Design review of the part built by this model. Coordinates are the model's own, in mm. Coordinates: 2 decimals unless noted, no trailing zeros. Order: outer loops, then holes, each group sorted by start corner. A loop starts at its lowest first (then second) coordinate and runs counter-clockwise, first axis right, second up. Notation, with made-up numbers: (37.25, 12.25) -> (84.25, 12.25) arc R11 cw to (84.25, 17.25) -> close; hole circle Ø8 at (-8.5, -14.75). An arc over 180 degrees is marked (long way). Use a Markdown table: item, result. Add a question column.
Q1. Insertion check: pin 1 (1.6 mm diameter, centred on x = -52, z = -2.5, fed in from -Y); pin 2 (1.6 mm diameter, centred on y = -15.5, z = -3, fed in from -X); pin 3 (8.5 mm diameter, centred on x = 0, y = 0, fed in from +Z); pin 4 (1.6 mm diameter, centred on x = 40.5, z = -3.5, fed in from +Y). Each pin has a flat end and moves straight along its axis. Give the tip position at first contact, or say it passes through.
Q2. Add section D-D (x = -30). State the section outline as (y, z) points, then the cut area to 3 significant figures.
Q3. Add section B-B (z = -2.9). Count the separate pieces of the cut face and the enclosed holes in it, then the cut area to 3 significant figures.
Q4. Add section A-A (x = 0). State the section outline as (y, z) points, then the cut area to 3 significant figures.
Q5. Wall thickness on probe 1 along X at (y, z) = (0, -3.05); probe 2 along Y at (x, z) = (30, -2.8); probe 3 along X at (y, z) = (21.5, -2.1): over which ranges is each line inside the solid? List them lowest first.
Q6. Add section C-C (y = 0). State the section outline as (x, z) points, then the cut area to 3 significant figures.
Autodesk Inventor part; units mm, degrees
ref_plane "YZ Plane" through (0, 0, 0) normal (1, 0, 0) x (0, 1, 0)
ref_plane "XZ Plane" through (0, 0, 0) normal (0, 1, 0) x (-1, 0, 0)
ref_plane "XY Plane" through (0, 0, 0) normal (0, 0, 1) x (1, 0, 0)
sketch "Block1" plane through (0, 0, 0) normal (0, 0, 1) x (1, 0, 0)
  line L0 (-37.5521, 20) -> (-37.5521, 24)
  line L1 (-37.5521, 24) -> (-17.5521, 24)
  line L2 (-17.5521, 24) -> (-17.5521, 20)
  line L3 (-37.4196, 20) -> (-17.5521, 20)
  line L4 (17.5521, 24) -> (17.5521, 20)
  line L5 (37.5521, 20) -> (37.5521, 24)
  line L6 (37.5521, 24) -> (17.5521, 24)
  line L7 (37.4196, 20) -> (17.5521, 20)
  point P0 (0, 21.8462)
  dimension "d140" = 20
  dimension "d141" = 4
sketch "Block2" plane through (0, 0, 0) normal (0, 0, 1) x (1, 0, 0)
  line L0 (-33.5533, 20.22) -> (-33.5533, 29.22)
  line L1 (-33.5533, 29.22) -> (-13.1133, 29.22)
  line L2 (-13.1133, 29.22) -> (-13.1133, 20.22)
  line L3 (-13.1133, 20.22) -> (13.1133, 20.22)
  line L4 (13.1133, 20.22) -> (13.1133, 29.22)
  line L5 (13.1133, 29.22) -> (33.5533, 29.22)
  line L6 (33.5533, 29.22) -> (33.5533, 20.22)
  line L7 (33.5533, 20.22) -> (50.22, 20.22)
  line L8 (50.22, 20.22) -> (50.22, 13.5533)
  line L9 (50.22, 13.5533) -> (59.22, 13.5533)
  line L10 (59.22, 13.5533) -> (59.22, 5.1133)
  line L11 (59.22, 5.1133) -> (50.22, 5.1133)
  line L12 (50.22, 5.1133) -> (50.22, -5.1133)
  line L13 (50.22, -5.1133) -> (59.22, -5.1133)
  line L14 (59.22, -5.1133) -> (59.22, -13.5533)
  line L15 (59.22, -13.5533) -> (50.22, -13.5533)
  line L16 (50.22, -13.5533) -> (50.22, -20.22)
  line L17 (50.22, -20.22) -> (-50.22, -20.22)
  line L18 (-50.22, -20.22) -> (-50.22, -13.5533)
  line L19 (-50.22, -13.5533) -> (-59.22, -13.5533)
  line L20 (-59.22, -13.5533) -> (-59.22, -5.1133)
  line L21 (-59.22, -5.1133) -> (-50.22, -5.1133)
  line L22 (-50.22, -5.1133) -> (-50.22, 5.1133)
  line L23 (-50.22, 5.1133) -> (-59.22, 5.1133)
  line L24 (-59.22, 5.1133) -> (-59.22, 13.5533)
  line L25 (-59.22, 13.5533) -> (-50.22, 13.5533)
  line L26 (-50.22, 13.5533) -> (-50.22, 20.22)
  line L27 (-50.22, 20.22) -> (-33.5533, 20.22)
  circle A0 centre (-30, 0) radius 4.72
  circle A1 centre (0, 0) radius 4.72
  circle A2 centre (30, 0) radius 4.72
  point P0 (0, 6.592)
sketch "Block3" plane through (0, 0, 0) normal (0, 0, 1) x (1, 0, 0)
  line L0 (-33.4333, 29.1) -> (-13.2333, 29.1)
  line L1 (-13.2333, 29.1) -> (-13.2333, 20.1)
  line L2 (-13.2333, 20.1) -> (13.2333, 20.1)
  line L3 (13.2333, 20.1) -> (13.2333, 29.1)
  line L4 (13.2333, 29.1) -> (33.4333, 29.1)
  line L5 (33.4333, 29.1) -> (33.4333, 20.1)
  line L6 (33.4333, 20.1) -> (50.1, 20.1)
  line L7 (50.1, 20.1) -> (50.1, 13.4333)
  line L8 (50.1, 13.4333) -> (59.1, 13.4333)
  line L9 (59.1, 13.4333) -> (59.1, 5.2333)
  line L10 (59.1, 5.2333) -> (50.1, 5.2333)
  line L11 (50.1, 5.2333) -> (50.1, -5.2333)
  line L12 (50.1, -5.2333) -> (59.1, -5.2333)
  line L13 (59.1, -5.2333) -> (59.1, -13.4333)
  line L14 (59.1, -13.4333) -> (50.1, -13.4333)
  line L15 (50.1, -13.4333) -> (50.1, -20.1)
  line L16 (50.1, -20.1) -> (-50.1, -20.1)
  line L17 (-50.1, -20.1) -> (-50.1, -13.4333)
  line L18 (-50.1, -13.4333) -> (-59.1, -13.4333)
  line L19 (-59.1, -13.4333) -> (-59.1, -5.2333)
  line L20 (-59.1, -5.2333) -> (-50.1, -5.2333)
  line L21 (-50.1, -5.2333) -> (-50.1, 5.2333)
  line L22 (-50.1, 5.2333) -> (-59.1, 5.2333)
  line L23 (-59.1, 5.2333) -> (-59.1, 13.4333)
  line L24 (-59.1, 13.4333) -> (-50.1, 13.4333)
  line L25 (-50.1, 13.4333) -> (-50.1, 20.1)
  line L26 (-50.1, 20.1) -> (-33.4333, 20.1)
  line L27 (-33.4333, 20.1) -> (-33.4333, 29.1)
  circle A0 centre (-30, 0) radius 5.6
  circle A1 centre (0, 0) radius 7.1
  circle A2 centre (30, 0) radius 5.6
  point P0 (0, 6.56)
sketch "Block4" plane through (0, 0, 0) normal (0, 0, 1) x (1, 0, 0)
  line L0 (-33.5333, 29.2) -> (-13.1333, 29.2)
  line L1 (-13.1333, 29.2) -> (-13.1333, 20.2)
  line L2 (-13.1333, 20.2) -> (13.1333, 20.2)
  line L3 (13.1333, 20.2) -> (13.1333, 29.2)
  line L4 (13.1333, 29.2) -> (33.5333, 29.2)
  line L5 (33.5333, 29.2) -> (33.5333, 20.2)
  line L6 (33.5333, 20.2) -> (50.2, 20.2)
  line L7 (50.2, 20.2) -> (50.2, 13.5333)
  line L8 (50.2, 13.5333) -> (59.2, 13.5333)
  line L9 (59.2, 13.5333) -> (59.2, 5.1333)
  line L10 (59.2, 5.1333) -> (50.2, 5.1333)
  line L11 (50.2, 5.1333) -> (50.2, -5.1333)
  line L12 (50.2, -5.1333) -> (59.2, -5.1333)
  line L13 (59.2, -5.1333) -> (59.2, -13.5333)
  line L14 (59.2, -13.5333) -> (50.2, -13.5333)
  line L15 (50.2, -13.5333) -> (50.2, -20.2)
  line L16 (50.2, -20.2) -> (-50.2, -20.2)
  line L17 (-50.2, -20.2) -> (-50.2, -13.5333)
  line L18 (-50.2, -13.5333) -> (-59.2, -13.5333)
  line L19 (-59.2, -13.5333) -> (-59.2, -5.1333)
  line L20 (-59.2, -5.1333) -> (-50.2, -5.1333)
  line L21 (-50.2, -5.1333) -> (-50.2, 5.1333)
  line L22 (-50.2, 5.1333) -> (-59.2, 5.1333)
  line L23 (-59.2, 5.1333) -> (-59.2, 13.5333)
  line L24 (-59.2, 13.5333) -> (-50.2, 13.5333)
  line L25 (-50.2, 13.5333) -> (-50.2, 20.2)
  line L26 (-50.2, 20.2) -> (-33.5333, 20.2)
  line L27 (-33.5333, 20.2) -> (-33.5333, 29.2)
  circle A0 centre (-30, 0) radius 5.7
  circle A1 centre (0, 0) radius 7.2
  circle A2 centre (30, 0) radius 5.7
  point P0 (0, 6.5867)
sketch "Block5" plane through (0, 0, 0) normal (0, 0, 1) x (1, 0, 0)
  line L0 (13.2333, 29.1) -> (33.4333, 29.1)
  line L1 (33.4333, 29.1) -> (33.4333, 20.1)
  line L2 (33.4333, 20.1) -> (50.1, 20.1)
  line L3 (50.1, 20.1) -> (50.1, 13.4333)
  line L4 (50.1, 13.4333) -> (59.1, 13.4333)
  line L5 (59.1, 13.4333) -> (59.1, 5.2333)
  line L6 (59.1, 5.2333) -> (50.1, 5.2333)
  line L7 (50.1, 5.2333) -> (50.1, -5.2333)
  line L8 (50.1, -5.2333) -> (59.1, -5.2333)
  line L9 (59.1, -5.2333) -> (59.1, -13.4333)
  line L10 (59.1, -13.4333) -> (50.1, -13.4333)
  line L11 (50.1, -13.4333) -> (50.1, -20.1)
  line L12 (50.1, -20.1) -> (-50.1, -20.1)
  line L13 (-50.1, -20.1) -> (-50.1, -13.4333)
  line L14 (-50.1, -13.4333) -> (-59.1, -13.4333)
  line L15 (-59.1, -13.4333) -> (-59.1, -5.2333)
  line L16 (-59.1, -5.2333) -> (-50.1, -5.2333)
  line L17 (-50.1, -5.2333) -> (-50.1, 5.2333)
  line L18 (-50.1, 5.2333) -> (-59.1, 5.2333)
  line L19 (-59.1, 5.2333) -> (-59.1, 13.4333)
  line L20 (-59.1, 13.4333) -> (-50.1, 13.4333)
  line L21 (-50.1, 13.4333) -> (-50.1, 20.1)
  line L22 (-50.1, 20.1) -> (-33.4333, 20.1)
  line L23 (-33.4333, 20.1) -> (-33.4333, 29.1)
  line L24 (-33.4333, 29.1) -> (-13.2333, 29.1)
  line L25 (-13.2333, 29.1) -> (-13.2333, 20.1)
  line L26 (-13.2333, 20.1) -> (13.2333, 20.1)
  line L27 (13.2333, 20.1) -> (13.2333, 29.1)
  circle A0 centre (-30, 0) radius 5.6
  circle A1 centre (0, 0) radius 7.1
  circle A2 centre (30, 0) radius 5.6
  point P0 (0, 6.56)
sketch "Block6" plane through (0, 0, 0) normal (0, 0, 1) x (1, 0, 0)
  line L0 (-33.4133, 25.58) -> (-13.2533, 25.58)
  line L1 (-13.2533, 25.58) -> (-13.2533, 20.08)
  line L2 (-13.2533, 20.08) -> (13.2533, 20.08)
  line L3 (13.2533, 20.08) -> (13.2533, 25.58)
  line L4 (13.2533, 25.58) -> (33.4133, 25.58)
  line L5 (33.4133, 25.58) -> (33.4133, 20.08)
  line L6 (33.4133, 20.08) -> (50.08, 20.08)
  line L7 (50.08, 20.08) -> (50.08, 13.4133)
  line L8 (50.08, 13.4133) -> (55.58, 13.4133)
  line L9 (55.58, 13.4133) -> (55.58, 5.2533)
  line L10 (55.58, 5.2533) -> (50.08, 5.2533)
  line L11 (50.08, 5.2533) -> (50.08, -5.2533)
  line L12 (50.08, -5.2533) -> (55.58, -5.2533)
  line L13 (55.58, -5.2533) -> (55.58, -13.4133)
  line L14 (55.58, -13.4133) -> (50.08, -13.4133)
  line L15 (50.08, -13.4133) -> (50.08, -20.08)
  line L16 (50.08, -20.08) -> (-50.08, -20.08)
  line L17 (-50.08, -20.08) -> (-50.08, -13.4133)
  line L18 (-50.08, -13.4133) -> (-55.58, -13.4133)
  line L19 (-55.58, -13.4133) -> (-55.58, -5.2533)
  line L20 (-55.58, -5.2533) -> (-50.08, -5.2533)
  line L21 (-50.08, -5.2533) -> (-50.08, 5.2533)
  line L22 (-50.08, 5.2533) -> (-55.58, 5.2533)
  line L23 (-55.58, 5.2533) -> (-55.58, 13.4133)
  line L24 (-55.58, 13.4133) -> (-50.08, 13.4133)
  line L25 (-50.08, 13.4133) -> (-50.08, 20.08)
  line L26 (-50.08, 20.08) -> (-33.4133, 20.08)
  line L27 (-33.4133, 20.08) -> (-33.4133, 25.58)
  circle A0 centre (-30, 0) radius 5.58
  circle A1 centre (0, 0) radius 7.08
  circle A2 centre (30, 0) radius 5.58
  point P0 (0, 6.088)
sketch "Block7" plane through (0, 0, 0) normal (0, 0, 1) x (1, 0, 0)
  line L0 (-33.4133, 25.58) -> (-13.2533, 25.58)
  line L1 (-13.2533, 25.58) -> (-13.2533, 20.08)
  line L2 (-13.2533, 20.08) -> (13.2533, 20.08)
  line L3 (13.2533, 20.08) -> (13.2533, 25.58)
  line L4 (13.2533, 25.58) -> (33.4133, 25.58)
  line L5 (33.4133, 25.58) -> (33.4133, 20.08)
  line L6 (33.4133, 20.08) -> (50.08, 20.08)
  line L7 (50.08, 20.08) -> (50.08, 13.4133)
  line L8 (50.08, 13.4133) -> (55.58, 13.4133)
  line L9 (55.58, 13.4133) -> (55.58, 5.2533)
  line L10 (55.58, 5.2533) -> (50.08, 5.2533)
  line L11 (50.08, 5.2533) -> (50.08, -5.2533)
  line L12 (50.08, -5.2533) -> (55.58, -5.2533)
  line L13 (55.58, -5.2533) -> (55.58, -13.4133)
  line L14 (55.58, -13.4133) -> (50.08, -13.4133)
  line L15 (50.08, -13.4133) -> (50.08, -20.08)
  line L16 (50.08, -20.08) -> (-50.08, -20.08)
  line L17 (-50.08, -20.08) -> (-50.08, -13.4133)
  line L18 (-50.08, -13.4133) -> (-55.58, -13.4133)
  line L19 (-55.58, -13.4133) -> (-55.58, -5.2533)
  line L20 (-55.58, -5.2533) -> (-50.08, -5.2533)
  line L21 (-50.08, -5.2533) -> (-50.08, 5.2533)
  line L22 (-50.08, 5.2533) -> (-55.58, 5.2533)
  line L23 (-55.58, 5.2533) -> (-55.58, 13.4133)
  line L24 (-55.58, 13.4133) -> (-50.08, 13.4133)
  line L25 (-50.08, 13.4133) -> (-50.08, 20.08)
  line L26 (-50.08, 20.08) -> (-33.4133, 20.08)
  line L27 (-33.4133, 20.08) -> (-33.4133, 25.58)
  circle A0 centre (-30, 0) radius 4.88
  circle A1 centre (0, 0) radius 7.08
  circle A2 centre (30, 0) radius 4.88
  point P0 (0, 6.088)
sketch "Sketch10" plane through (0, 0, 0) normal (0, 0, 1) x (1, 0, 0)
  line L0 (50, -20) -> (-50, -20)
  line L1 (-50, -20) -> (-50, 20)
  line L2 (-50, 20) -> (50, 20)
  line L3 (50, 20) -> (50, -20)
  line L4 (50, -20) -> (-50, 20) construction
  line L5 (-50, -20) -> (50, 20) construction
  point P0 (0, 0)
  dimension "d21" = 100
  dimension "d22" = 40
extrude "Extrusion2" add sketch "Sketch10" against normal blind 5.5
sketch "Sketch16" plane through (0, 0, -5.5) normal (0, 0, -1) x (-1, 0, 0)
  line L0 (0, -30.0399) -> (0, 39.5395)
  point P0 (0, 0)
  point P1 (-30, 0)
  point P2 (30, 0)
  dimension "d52" = 60
hole "Hole5" at (30, 0, -5.5) at (-30, 0, -5.5) direction (0, 0, 1) diameter 9.6 end through all
sketch "Sketch17" plane through (0, 0, -5.5) normal (0, 0, -1) x (-1, 0, 0)
  point P0 (0, 0)
  point P1 (0, 0)
hole "Hole14" at (0, 0, -5.5) direction (0, 0, 1) diameter 14 end through all
sketch "Sketch34" plane through (0, 0, 0) normal (0, 0, 1) x (1, 0, 0)
  line L0 (-50, 20) -> (50, 20)
  line L1 (-50, -20) -> (-50, 20)
  line L2 (-30, 20) -> (-10, 20)
  line L3 (0, -30.0399) -> (0, 39.5395)
  line L4 (-234.7041, 0) -> (108.0673, 0)
  line L5 (-30, 20) -> (-30, 25.5)
  line L6 (-10, 20) -> (-10, 25.5)
  line L7 (-10, 25.5) -> (-30, 25.5)
  line L8 (30, 20) -> (10, 20)
  line L9 (30, 20) -> (30, 25.5)
  line L10 (10, 20) -> (10, 25.5)
  line L11 (10, 25.5) -> (30, 25.5)
  line L12 (-50, 13.3333) -> (-55.5, 13.3333)
  line L13 (-55.5, 13.3333) -> (-55.5, 5.3333)
  line L14 (-55.5, 5.3333) -> (-50, 5.3333)
  line L15 (-50, 13.3333) -> (-50, 5.3333)
  line L16 (50, 13.3333) -> (55.5, 13.3333)
  line L17 (55.5, 13.3333) -> (55.5, 5.3333)
  line L18 (55.5, 5.3333) -> (50, 5.3333)
  line L19 (50, 13.3333) -> (50, 5.3333)
  line L20 (-50, -13.3333) -> (-55.5, -13.3333)
  line L21 (-55.5, -13.3333) -> (-55.5, -5.3333)
  line L22 (-55.5, -5.3333) -> (-50, -5.3333)
  line L23 (-50, -13.3333) -> (-50, -5.3333)
  line L24 (50, -13.3333) -> (50, -5.3333)
  line L25 (55.5, -13.3333) -> (55.5, -5.3333)
  line L26 (55.5, -5.3333) -> (50, -5.3333)
  line L27 (50, -13.3333) -> (55.5, -13.3333)
  dimension "d131" = 20
  dimension "d132" = 5.5
  dimension "d133" = 5.5
  dimension "d134" = 8
  dimension "d135" = 6.6667
extrude "Extrusion4" add sketch "Sketch34" against normal blind 5.5 contours L1 L20 L21 L22 | L1 L14 L13 L12 | L16 L17 L18 L19 | L24 L26 L25 L27
sketch "Sketch35" plane through (0, 0, 0) normal (0, 0, 1) x (1, 0, 0)
  line L0 (-50, 20) -> (50, 20)
  line L1 (-50, 13.3333) -> (-50, 20)
  line L2 (0, -30.0399) -> (0, 39.5395)
  line L3 (-33.3333, 20) -> (-13.3333, 20)
  line L4 (-13.3333, 20) -> (-13.3333, 25.5)
  line L5 (-13.3333, 25.5) -> (-33.3333, 25.5)
  line L6 (-33.3333, 25.5) -> (-33.3333, 20)
  line L7 (33.3333, 20) -> (13.3333, 20)
  line L8 (13.3333, 20) -> (13.3333, 25.5)
  line L9 (13.3333, 25.5) -> (33.3333, 25.5)
  line L10 (33.3333, 25.5) -> (33.3333, 20)
  dimension "d142" = 16.6667
  dimension "d143" = 20
  dimension "d144" = 5.5
extrude "Extrusion5" add sketch "Sketch35" against normal blind 5.5
equation "\"d140\" = 0.2 * d21"
equation "\"d141\" = At"
equation "\"d23\" = Wt"
equation "\"d131\" = 0.2 * d21"
equation "\"d132\" = Wt"
equation "\"d133\" = Wt"
equation "\"d134\" = 0.2 * d22"
equation "\"d135\" = 0.166667 * d22"
equation "\"d138\" = Wt"
equation "\"d142\" = 0.166667 * d21"
equation "\"d143\" = 0.2 * d21"
equation "\"d144\" = Wt"
equation "\"d145\" = Wt"
properties part number "holder_plate" material "Wood (Birch)"
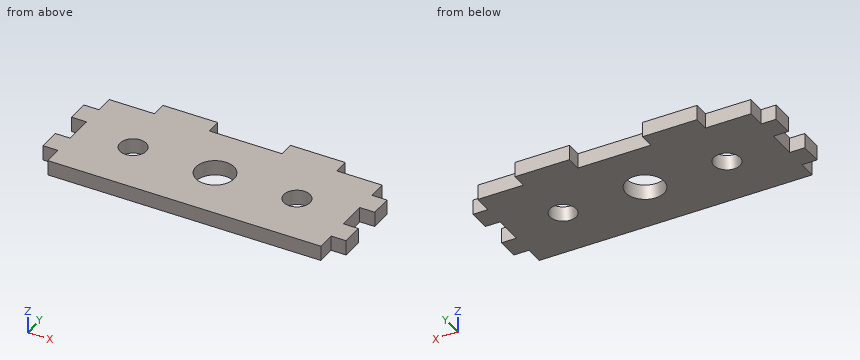
Established:
| question | item | result |
|---|---|---|
| 1 | pin 1 | y = -13.33 |
| 1 | pin 2 | x = -50 |
| 1 | pin 3 | through |
| 1 | pin 4 | y = 20 |
| 2 | outline | (-20, -5.5) -> (-4.8, -5.5) -> (-4.8, 0) -> (-20, 0) -> close; (4.8, -5.5) -> (25.5, -5.5) -> (25.5, 0) -> (4.8, 0) -> close |
| 2 | area | 197 mm^2 |
| 3 | separate pieces | 1 |
| 3 | enclosed holes | 3 |
| 3 | area | 4,100 mm^2 |
| 4 | outline | (-20, -5.5) -> (-7, -5.5) -> (-7, 0) -> (-20, 0) -> close; (7, -5.5) -> (20, -5.5) -> (20, 0) -> (7, 0) -> close |
| 4 | area | 143 mm^2 |
| 5 | probe 1 | -50 to -34.8, -25.2 to -7, 7 to 25.2, 34.8 to 50 |
| 5 | probe 2 | -20 to -4.8, 4.8 to 25.5 |
| 5 | probe 3 | -33.33 to -13.33, 13.33 to 33.33 |
| 6 | outline | (-50, -5.5) -> (-34.8, -5.5) -> (-34.8, 0) -> (-50, 0) -> close; (-25.2, -5.5) -> (-7, -5.5) -> (-7, 0) -> (-25.2, 0) -> close; (7, -5.5) -> (25.2, -5.5) -> (25.2, 0) -> (7, 0) -> close; (34.8, -5.5) -> (50, -5.5) -> (50, 0) -> (34.8, 0) -> close |
| 6 | area | 367 mm^2 |
